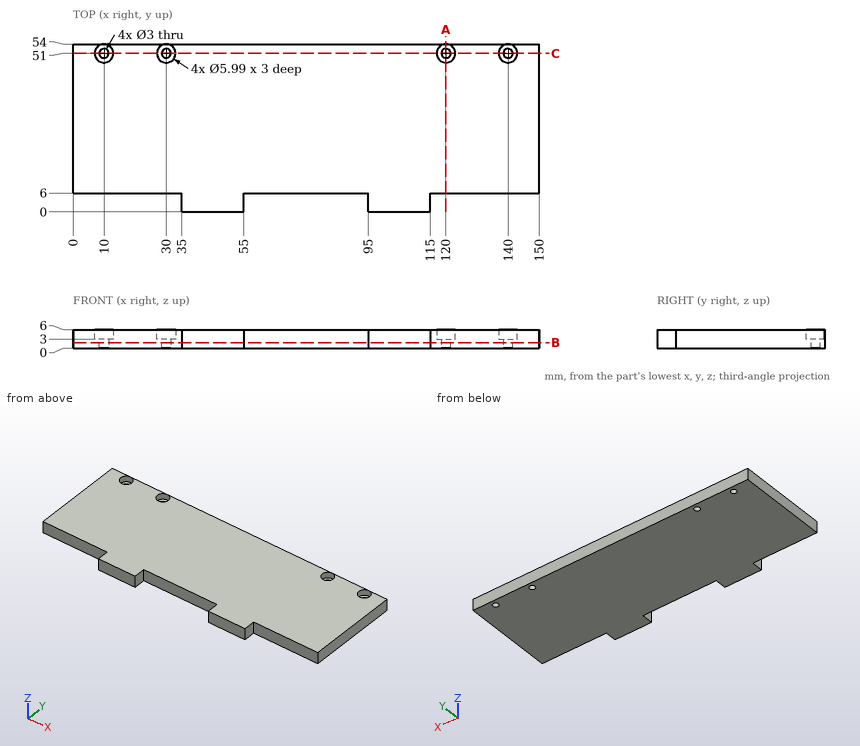
Answer from the drawing. Dimensions are ordinates in mm from the lowest x, y and z of the part. Give positions to 0.01 mm unless a question says otherwise; leave off trailing zeros. Write each loop counter-clockwise with the first axis right and the second up, starting at its lowest first coordinate (ties: lowest second). Pieces come first, ordered by that corner, then holes.
1) Section A-A (x = 120) is taken. Write down the section's boundary in (y, z) (3 decimals), and give its area (3 significant figures).
2) Section B-B (z = 1.9) is taken. Write down the section's boundary in (x, y), and give its area (3 significant figures).
3) Given P1, Ø3.5, axis at x = 30, y = 51, coming from the +Z side; P2, Ø3, axis at y = 2.5, z = 3, coming from the +X side; P3, Ø3, axis at x = 17, z = 3, coming from the -Y side, each flat-ended and moving along its own axis, determine where each tip first touches the part or whether it passes through.
4) Section C-C (y = 51) is taken. Count the separate pieces of the cut face and the enclosed holes in it, and give its area (3 significant figures).
5) Find the intervals of material crossed by L1, parallel to X at y = 5.5, z = 3.8; L2, parallel to X at y = 49, z = 3.55; L3, parallel to Y at x = 10, z = 1.25, in increasing order.
Response:
1. outline: (6, 0) - (49.5, 0) - (49.5, 3) - (48.005, 3) - (48.005, 6) - (6, 6) - close; (52.5, 0) - (54, 0) - (54, 6) - (53.995, 6) - (53.995, 3) - (52.5, 3) - close
1. area: 261 mm2
2. outline: (0, 6) - (35, 6) - (35, 0) - (55, 0) - (55, 6) - (95, 6) - (95, 0) - (115, 0) - (115, 6) - (150, 6) - (150, 54) - (0, 54) - close; hole circle Ø3 at (10, 51); hole circle Ø3 at (30, 51); hole circle Ø3 at (120, 51); hole circle Ø3 at (140, 51)
2. area: 7,410 mm2
3. P1: stops at z = 3
3. P2: stops at x = 115
3. P3: stops at y = 6
4. separate pieces: 5
4. enclosed holes: 0
4. area: 792 mm2
5. L1: x = 35 to 55, 95 to 115
5. L2: x = 0 to 7.77, 12.23 to 27.77, 32.23 to 117.77, 122.23 to 137.77, 142.23 to 150
5. L3: y = 6 to 49.5, 52.5 to 54
